For this review, take the finished solid that the model builds, in its own axes (mm). Give positions to 0.01 mm unless a question says otherwise; leave off trailing zeros. Order: outer loops, then holes, each group sorted by start corner. A loop starts at its lowest first (then second) coordinate and runs counter-clockwise, first axis right, second up. Notation, with made-up numbers: M 6,-3.75 L 41,-3.75 A29 cw 41,29.25 Z; hole C -20,0 d11. An arc over 180 degrees is marked long. Use CSV: the item, a comma, the result in double quotes. Start each with the question number.
(1) Consider section D-D (z = 2). Write out the cut boundary in (x, y).
(2) Consider section B-B (y = 226). Write out the cut boundary in (x, z).
(3) Wall thickness on L1, parallel to X at y = 82, z = 1.25; L2, parallel to Y at x = 87, z = 4.5; L3, parallel to X at y = 98, z = 5.75: over which ranges is each line inside the solid? List them lowest first. Write a range as from..to.
(4) Consider section C-C (x = 98.5). Write out the cut boundary in (y, z).
(5) Consider section A-A (x = 59). Write out the cut boundary in (y, z).
(6) Clearance check with a flat-ended pin moving along its axis: P1, Ø1.5, axis at x = 100, z = 1.5, coming from the -Y side. State where the tip first meets the part, or that it passes through.
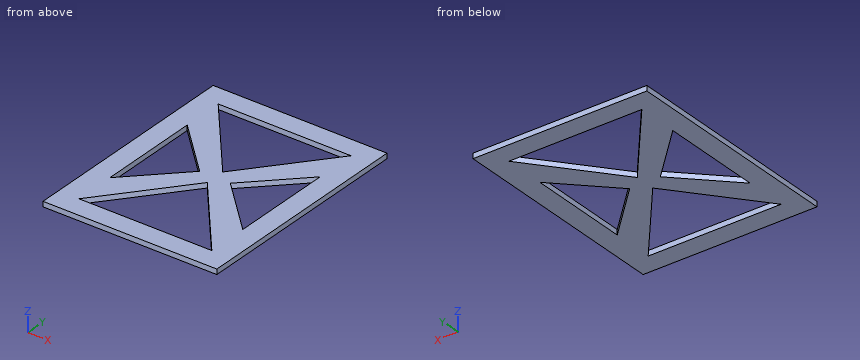
```python
from build123d import *

# Parameters (mm, degrees)
F0_W     = 215.9
F0_H     = 279.4
F1_DEPTH = 6.35


with BuildPart() as f1:
    # F0 (on Top) → F1 (new body)
    with BuildSketch(Plane.XY):
        with Locations((112.702514, 139.7)):
            Rectangle(F0_W, F0_H)
        Polygon((30.152514, 25.4), (112.702514, 127), (195.252514, 25.4), align=None, mode=Mode.SUBTRACT)
        Polygon((30.152514, 76.2), (30.152514, 203.2), (93.652514, 139.7), align=None, mode=Mode.SUBTRACT)
        Polygon((112.702514, 152.4), (30.152514, 254), (195.252514, 254), align=None, mode=Mode.SUBTRACT)
        Polygon((195.252514, 76.2), (131.752514, 139.7), (195.252514, 203.2), align=None, mode=Mode.SUBTRACT)
    extrude(amount=F1_DEPTH)


solid = f1.part
```
Check result:
1,outline,"M 4.75,0 L 220.65,0 L 220.65,279.4 L 4.75,279.4 Z; hole M 30.15,25.4 L 195.25,25.4 L 112.7,127 Z; hole M 30.15,76.2 L 93.65,139.7 L 30.15,203.2 Z; hole M 30.15,254 L 112.7,152.4 L 195.25,254 Z; hole M 131.75,139.7 L 195.25,76.2 L 195.25,203.2 Z"
2,outline,"M 4.75,0 L 52.9,0 L 52.9,6.35 L 4.75,6.35 Z; M 172.5,0 L 220.65,0 L 220.65,6.35 L 172.5,6.35 Z"
3,L1,"x = 4.75..30.15, 35.95..76.14, 149.27..189.45, 195.25..220.65"
3,L2,"y = 0..25.4, 95.37..133.05, 146.35..184.03, 254..279.4"
3,L3,"x = 4.75..30.15, 51.95..89.14, 136.27..173.45, 195.25..220.65"
4,outline,"M 0,0 L 25.4,0 L 25.4,6.35 L 0,6.35 Z; M 109.52,0 L 169.88,0 L 169.88,6.35 L 109.52,6.35 Z; M 254,0 L 279.4,0 L 279.4,6.35 L 254,6.35 Z"
5,outline,"M 0,0 L 25.4,0 L 25.4,6.35 L 0,6.35 Z; M 60.9,0 L 105.05,0 L 105.05,6.35 L 60.9,6.35 Z; M 174.35,0 L 218.5,0 L 218.5,6.35 L 174.35,6.35 Z; M 254,0 L 279.4,0 L 279.4,6.35 L 254,6.35 Z"
6,P1,"stops at y = 0"
